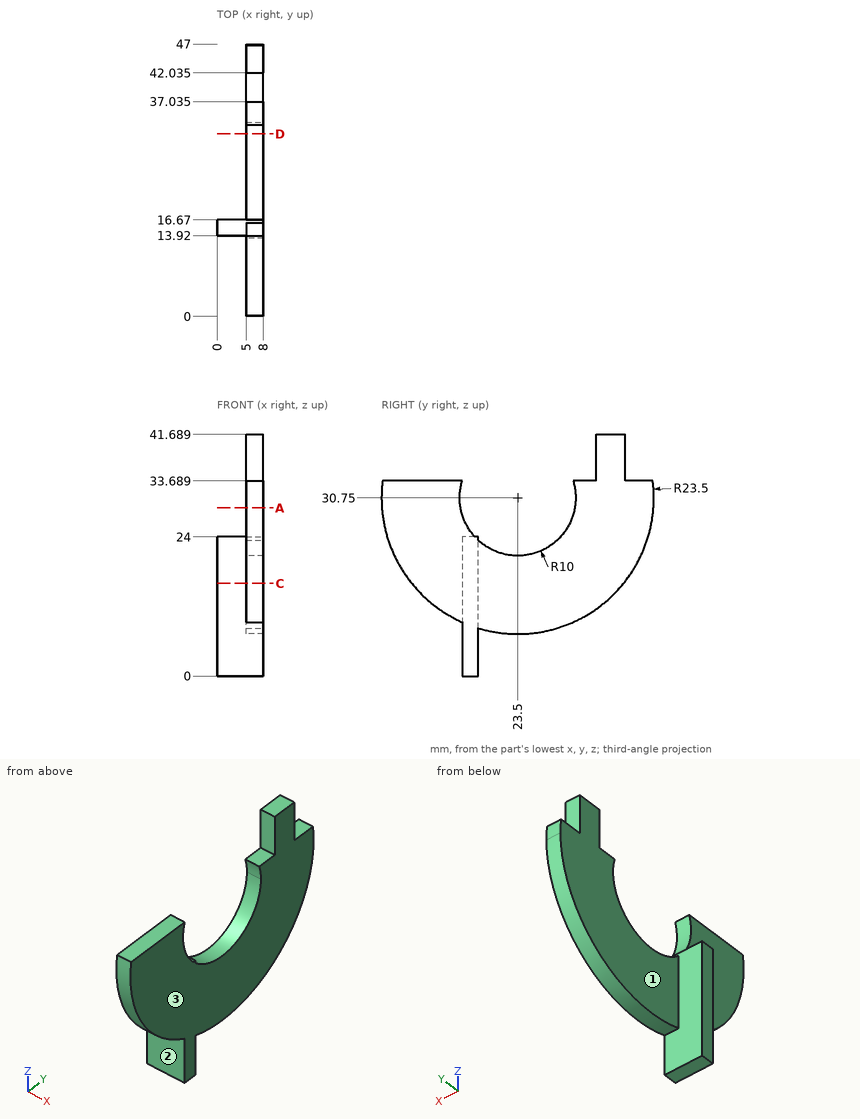
Geometry: see drawing. Coordinates: mm, zero at the bounding-box minimum. A direction names the side the tool comes from. Give positions to 0.01 mm unless a question says otherwise; leave off trailing zeros. Order: outer loops, then holes, each group sorted by start corner. A loop starts at its lowest first (then second) coordinate and runs counter-clockwise, first axis right, second up. Notation, with made-up numbers: (42.25, 56) -> (90.25, 56) arc R8 ccw to (90.25, 67) -> close; hole circle Ø3 at (35, -33.5). An arc over 180 degrees is marked (long way). Write item = value, one per line.
Q1. Cut plane A-A, the plane z = 29. Output: boundary loops of the cut face in (x, y) (1 decimal).
Data:
outline = (5, 0.1) -> (8, 0.1) -> (8, 13.7) -> (5, 13.7) -> close; (5, 33.3) -> (8, 33.3) -> (8, 46.9) -> (5, 46.9) -> close
Q2. Cut plane C-C, the plane z = 16. Output: boundary loops of the cut face in (x, y) (1 decimal).
Data:
outline = (0, 13.9) -> (5, 13.9) -> (5, 5.2) -> (8, 5.2) -> (8, 41.8) -> (5, 41.8) -> (5, 16.7) -> (0, 16.7) -> close
Q3. Material intervals for line 1 (Y direction, x = 5.75, z = 35) (1 decimal); line 2 (Y direction, x = 3.5, z = 23); line 3 (Z direction, x = 4, y = 14), sorted ascending. Write a range as from..to.
Data:
line_1 = 37..42
line_2 = 13.92..16.67
line_3 = 0..24
Q4. Cut plane D-D, the plane y = 31.5. Output: boundary loops of the cut face in (x, z), and give its area (3 significant figures).
Data:
outline = (5, 8.65) -> (8, 8.65) -> (8, 24.75) -> (5, 24.75) -> close
area = 48.3 mm^2
Q5. Pin query (flat end, axial travel): pin 1 (15 mm diameter, centred on y = 27, z = 18, fed in from -X); pin 2 (1.5 mm diameter, centred on x = 6, y = 35, fed in from +Z); pin 3 (4 mm diameter, centred on x = 4, z = 8.5, fed in from +Y) (1 decimal). Return the tip coordinate at first contact, or that it passes through.
Data:
pin_1 = 5
pin_2 = 33.69
pin_3 = 35
Q6. Set-up query: the marked faces 1, 2 and 3. Return all of +Z, -Z, +X, -X, +Y, -Y with unobstructed straight access to the full face (end or side cutting, diameter ignored); none if empty.
Data:
face_1 = +Z, -Z, -X, +Y
face_2 = -Z, -X, -Y
face_3 = +Z, -Z, +X, +Y, -Y
